Part model, mm, in its own coordinate system. A direction names the side the tool comes from. Give positions to 0.01 mm unless a question says otherwise; leave off trailing zeros. Write each loop counter-clockwise with the first axis right and the second up, starting at its lowest first coordinate (ties: lowest second). Pieces come first, ordered by that corner, then holes.
Autodesk Inventor part; units mm, degrees
ref_plane "YZ Plane" through (0, 0, 0) normal (1, 0, 0) x (0, 1, 0)
ref_plane "XZ Plane" through (0, 0, 0) normal (0, 1, 0) x (-1, 0, 0)
ref_plane "XY Plane" through (0, 0, 0) normal (0, 0, 1) x (1, 0, 0)
sketch "Sketch1" plane through (0, 0, 0) normal (0, 0, 1) x (1, 0, 0)
  line L0 (-46, -200) -> (46, -200)
  line L1 (46, -200) -> (46, 200)
  line L2 (46, 200) -> (-46, 200)
  line L3 (-46, 200) -> (-46, -200)
  line L4 (-46, -200) -> (46, 200) construction
  line L5 (46, -200) -> (-46, 200) construction
  point P0 (0, 0)
  dimension "d154" = 92
  dimension "d155" = 400
extrude "Plate5" add sketch "Sketch1" along normal blind 2
sketch "Sketch7" plane through (-44, -200, 0) normal (-1, 0, 0) x (0, -1, 0)
  line L0 (-400, 0) -> (0, 0)
  line L1 (0, 0) -> (0, 94)
  line L2 (0, 94) -> (-400, 94)
  line L3 (-400, 94) -> (-400, 0)
edge flange "Flange3" height 94 angle 90 thickness 2 bend radius 2.75 thickness toward (-1, 0, 0) relief round relief width 2 relief depth 1 edges at (-46, 0, 2) wall of the first edge with corners at (-44, 200, 0) (-44, -200, 0) (-44, -200, 94) (-44, 200, 94)
bend "Bend3"
corner "Corner3"
sketch "Sketch8" plane through (0, 0, 2) normal (0, 0, 1) x (1, 0, 0)
  line L0 (46, 200) -> (46, -200)
  line L1 (-41.25, 200) -> (46, 200)
  line L2 (32.375, 195) -> (-27.625, 195)
  line L3 (-27.625, 195) -> (-27.625, 125)
  line L4 (-27.625, 125) -> (32.375, 125)
  line L5 (32.375, 125) -> (32.375, 195)
  line L6 (32.375, 195) -> (-27.625, 125) construction
  line L7 (-27.625, 195) -> (32.375, 125) construction
  point P0 (0, 0)
  point P1 (2.375, 160)
  point P2 (2.375, 200)
  dimension "d167" = 60
  dimension "d168" = 70
  dimension "d169" = 5
extrude "Cut1" cut sketch "Sketch8" against normal blind 2
properties part number "PNS 752 FDS 1200 FLANGE 2" material "Stainless Steel"
1) Saw through at C-C (y = -55). Write the cut outline in (x, z), and give its area (3 significant figures).
Check result:
outline: (-46, 4.75) arc R4.75 ccw to (-41.25, 0) - (46, 0) - (46, 2) - (-41.25, 2) arc R2.75 cw to (-44, 4.75) - (-44, 94) - (-46, 94) - close
area: 365 mm2
2) Saw through at B-B (y = 141). Write the cut outline in (x, z) (3 decimals).
Check result:
outline: (-46, 4.75) arc R4.75 ccw to (-41.25, 0) - (-27.625, 0) - (-27.625, 2) - (-41.25, 2) arc R2.75 cw to (-44, 4.75) - (-44, 94) - (-46, 94) - close; (32.375, 0) - (46, 0) - (46, 2) - (32.375, 2) - close
3) 3-axis set-ups, long thin cutter, end or side, ignore diameter. For faces 1 (the flat face through (-45, -200, 26)), 2 (the flat face through (-44, -3, 49)): which of +Z, -Z, +X, -X, +Y, -Y reach the whole face in a straight line?
Check result:
face 1: +Z, -Z, +X, -X, -Y
face 2: +Z, +X, +Y, -Y
4) Saw through at D-D (z = 26). Write the cut outline in (x, y).
Check result:
outline: (-46, -200) - (-44, -200) - (-44, 200) - (-46, 200) - close
5) Flat gauge pins, fed straight in: P1, Ø2, axis at y = 148, z = 0.5, coming from the -X side; P2, Ø10, axis at x = -31, y = 65.5, coming from the +Z side; P3, Ø6, axis at y = 106.5, z = 25, coming from the +X side. Where does each tip first touch, or does it go through?
Check result:
P1: stops at x = -44.71
P2: stops at z = 2
P3: stops at x = -44
6) Saw through at A-A (x = 26). Write the cut outline in (y, z).
Check result:
outline: (-200, 0) - (125, 0) - (125, 2) - (-200, 2) - close; (195, 0) - (200, 0) - (200, 2) - (195, 2) - close
7) Drill centre lines: L1, parallel to Z at x = 21.5, y = 76; L2, parallel to X at y = -58, z = 56. Where is each one in solid material? Low to high.
Check result:
L1: z = 0 to 2
L2: x = -46 to -44
